from build123d import *

# Parameters (mm, degrees)
SKETCH_1_W      = 42
SKETCH_1_H      = 42
SKETCH_1_R      = 12.5
SKETCH_1_R_2    = 1.7
EXTRUDE_1_DEPTH = 5
FILLET_1_R      = 7


with BuildPart() as part:
    # 草图1 → 凸台-拉伸1 (new body)
    with BuildSketch(Plane.XY):
        Rectangle(SKETCH_1_W, SKETCH_1_H)
        Circle(SKETCH_1_R, mode=Mode.SUBTRACT)
        with Locations((-15.5, -15.5)):
            Circle(SKETCH_1_R_2, mode=Mode.SUBTRACT)
        with Locations((15.5, -15.5)):
            Circle(SKETCH_1_R_2, mode=Mode.SUBTRACT)
        with Locations((15.5, 15.5)):
            Circle(SKETCH_1_R_2, mode=Mode.SUBTRACT)
        with Locations((-15.5, 15.5)):
            Circle(SKETCH_1_R_2, mode=Mode.SUBTRACT)
    extrude(amount=EXTRUDE_1_DEPTH)

    # 圆角1
    fillet_1_edges = [part.edges().sort_by_distance(p)[0] for p in [
        (21, -21, 2.5),
        (-21, -21, 2.5),
        (-21, 21, 2.5),
        (21, 21, 2.5),
    ]]
    fillet(fillet_1_edges, radius=FILLET_1_R)


solid = part.part
Could you check a few things on this model? Use its own coordinates, in mm. Give positions to 0.01 mm unless a question says otherwise; leave off trailing zeros. Order: outer loops, then holes, each group sorted by start corner. A loop starts at its lowest first (then second) coordinate and runs counter-clockwise, first axis right, second up. Notation, with made-up numbers: M 89.25,-14.5 L 98.25,-14.5 A9 ccw 98.25,-1.5 Z; hole C 18.25,71.25 d6. An arc over 180 degrees is marked long. One line per question, with ' | ' between items.
1. If I drill on line 1 (Y direction, x = 15.5, z = 3.1); line 2 (Y direction, x = 16, z = 2.05); line 3 (X direction, y = 17, z = 4.05), over which ranges is the centre line in solid material (lowest first)?
Results:
line 1: -20.84 to -17.2, -13.8 to 13.8, 17.2 to 20.84 | line 2: -20.71 to -17.12, -13.88 to 13.88, 17.12 to 20.71 | line 3: -20.32 to -16.3, -14.7 to 14.7, 16.3 to 20.32
2. I want a section at A-A (z = 2.9). List the corners of the cut face in (x, y) for me.
Results:
outline: M -21,-14 A7 ccw -14,-21 L 14,-21 A7 ccw 21,-14 L 21,14 A7 ccw 14,21 L -14,21 A7 ccw -21,14 Z; hole C -15.5,-15.5 d3.4; hole C -15.5,15.5 d3.4; hole C 0,0 d25; hole C 15.5,-15.5 d3.4; hole C 15.5,15.5 d3.4
3. I want a section at B-B (x = 0). List the corners of the cut face in (y, z) for me.
Results:
outline: M -21,0 L -12.5,0 L -12.5,5 L -21,5 Z; M 12.5,0 L 21,0 L 21,5 L 12.5,5 Z
4. We'd pull the mould along Y, two halves only. Please class faces 1 (the face through (-21, 0, 2)), 2 (the face through (-19, -18.9, 2.5)), 3 (the face through (-14.7, 14, 2.5)): +Y half, -Y half, draft (parallel to the pull), parting line (faces both ways), or undercut.
Results:
face 1: draft | face 2: -Y half | face 3: undercut
5. I want a section at C-C (y = 15.5). List the corners of the cut face in (x, z) for me, and give its area (3 significant figures).
Results:
outline: M -20.84,0 L -17.2,0 L -17.2,5 L -20.84,5 Z; M -13.8,0 L 13.8,0 L 13.8,5 L -13.8,5 Z; M 17.2,0 L 20.84,0 L 20.84,5 L 17.2,5 Z | area: 174 mm²
6. I'm going to push a flat-ended pin straight in: pin 1 (22.5 mm diameter, centred on x = 0, y = 0, fed in from -Z). Where does the tip first touch, or does it pass through?
Results:
pin 1: through
